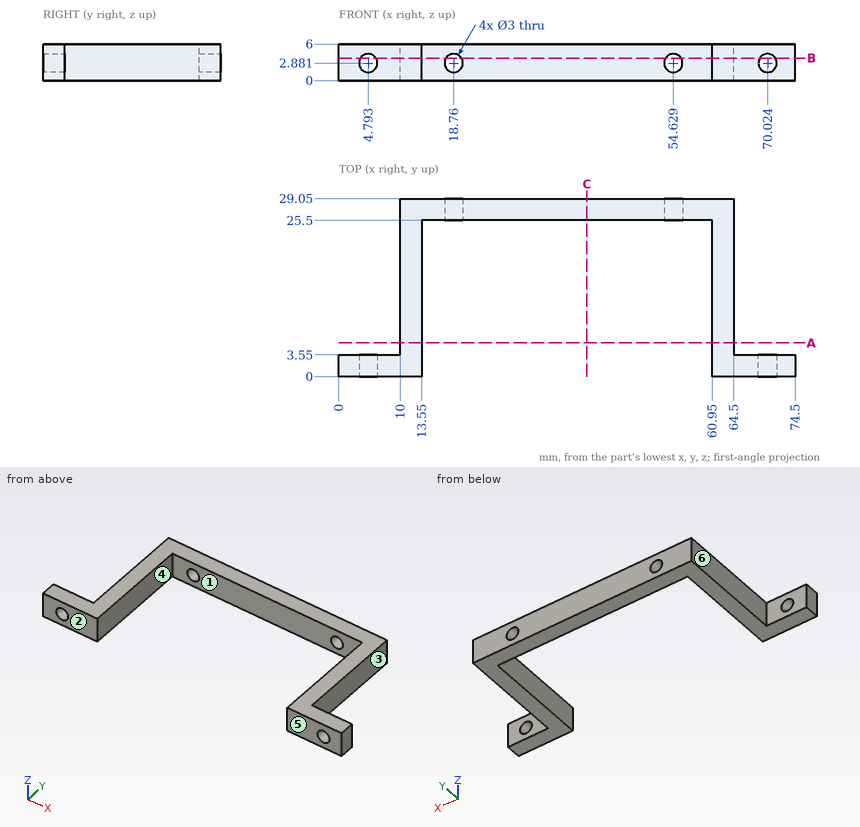
Verification items for this drawing (mm, ordinates from the low corner). A direction names the side the tool comes from. Coordinates: 2 decimals unless noted, no trailing zeros. Loops run counter-clockwise (first coordinate to the right, second up) from the corner with the lowest first, then second, coordinate; pieces in that order, holes last. Notation, with made-up numbers: (17.25, 63) - (72.25, 63) arc R20 ccw to (72.25, 67) - close; hole circle Ø9 at (-32, 46). An arc over 180 degrees is marked (long way). Answer as a JSON object with one key per item and string values.
(1) Cross-section at C-C, the plane x = 40.5. Record the boundary of the cut face in (y, z), then the cut area to 3 significant figures.
Response:
{"outline": "(25.5, 0) - (29.05, 0) - (29.05, 6) - (25.5, 6) - close", "area": "21.3 mm²"}
(2) Mould release check, pull along X, two halves, no side actions. Record for the marked faces 1, 2 and 3: pulls with the +X half, pulls with the -X half, needs draft (parallel to the pull), parting line crosses it, or undercut.
Response:
{"face 1": "undercut", "face 2": "needs draft", "face 3": "pulls with the +X half"}
(3) Cross-section at A-A, the plane y = 5.5. Record the boundary of the cut face in (x, z).
Response:
{"outline": "(10, 0) - (13.55, 0) - (13.55, 6) - (10, 6) - close; (60.95, 0) - (64.5, 0) - (64.5, 6) - (60.95, 6) - close"}
(4) Go/stop test with flat-tipped pins: pin 1 Ø1.8 at (y, z) = (18.5, 4) entering from +X; pin 2 Ø3 at (y, z) = (16, 4.5) entering from -X; pin 3 Ø3 at (x, z) = (24.5, 4) entering from -Y. Record where each tip stops, or that it passes through.
Response:
{"pin 1": "stops at x = 64.5", "pin 2": "stops at x = 10", "pin 3": "stops at y = 25.5"}
(5) Cross-section at B-B, the plane z = 3.7. Record the boundary of the cut face in (x, y).
Response:
{"outline": "(0, 0) - (3.54, 0) - (3.54, 3.55) - (0, 3.55) - close; (6.05, 0) - (13.55, 0) - (13.55, 25.5) - (17.5, 25.5) - (17.5, 29.05) - (10, 29.05) - (10, 3.55) - (6.05, 3.55) - close; (20.02, 25.5) - (53.37, 25.5) - (53.37, 29.05) - (20.02, 29.05) - close; (55.89, 25.5) - (60.95, 25.5) - (60.95, 0) - (68.77, 0) - (68.77, 3.55) - (64.5, 3.55) - (64.5, 29.05) - (55.89, 29.05) - close; (71.28, 0) - (74.5, 0) - (74.5, 3.55) - (71.28, 3.55) - close"}
(6) Scan lines: line 1 along X through (y, z) = (18.5, 1.2); line 2 along X through (y, z) = (26.5, 2.55); line 3 along Y through (x, z) = (68, 5.2). Record each from-to range of solid material in increasing order.
Response:
{"line 1": "x = 10 to 13.55, 60.95 to 64.5", "line 2": "x = 10 to 17.3, 20.22 to 53.17, 56.09 to 64.5", "line 3": "y = 0 to 3.55"}
(7) Access from +Z, -Z, +X, -X, +Y, -Y to the whole of each face (thin tool, end or side, straight path). Record for the marked faces 4, 5 and 6.
Response:
{"face 4": "+Z, -Z, -Y", "face 5": "+Z, -Z, +X, -X, -Y", "face 6": "+Z, -Z, -X, +Y"}
